For this review, use the dimensioned drawing (mm, ordinates from the lowest corner) and the shaded views. Round coordinates to 2 decimals unless told otherwise and drop trailing zeros. Write each loop counter-clockwise with the first axis right and the second up, starting at its lowest first coordinate (ties: lowest second). Pieces come first, ordered by that corner, then holes. Notation, with made-up numbers: M 47.5,46 L 99.5,46 A20 ccw 99.5,63 Z; hole C 74.25,72 d11. An arc over 180 degrees is marked long. One line per question, with ' | ' between items.
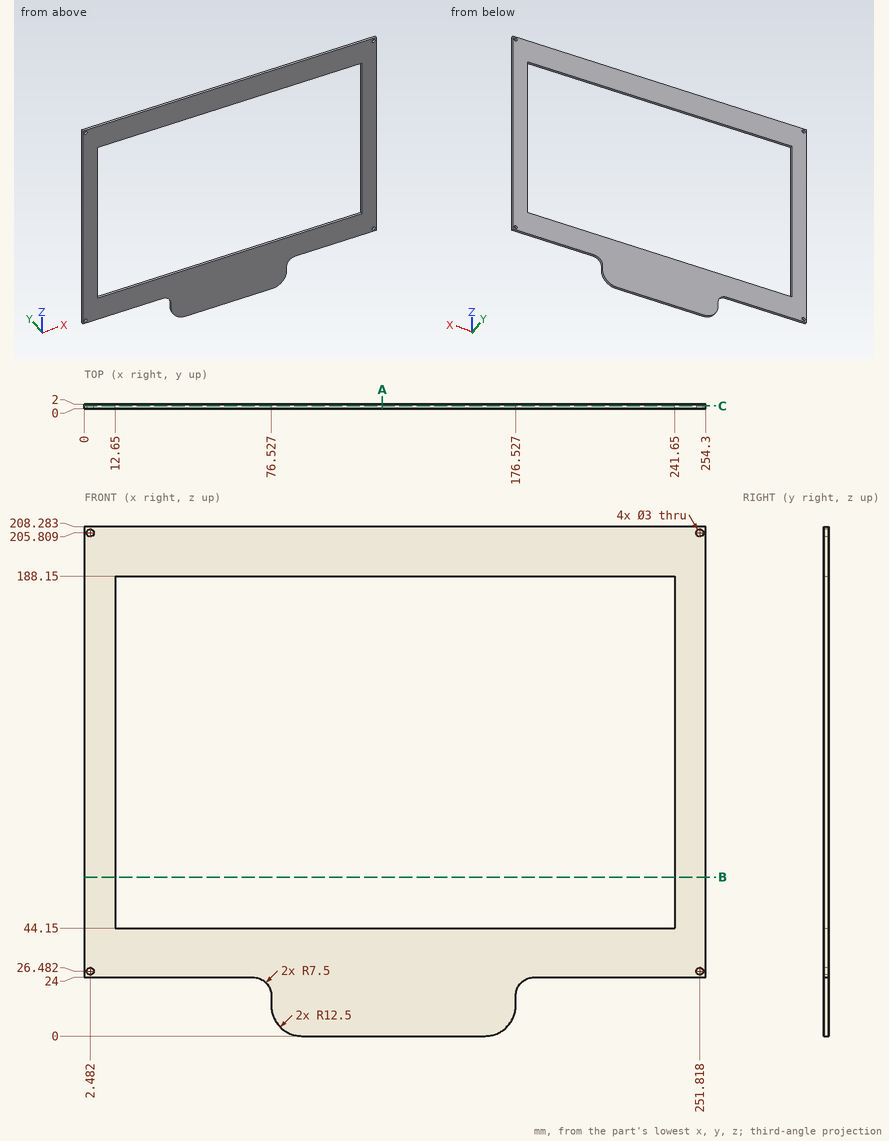
Item 1: Take a section at C-C (y = 1.2). Write out the cut boundary in (x, z).
Results:
outline: M 0,24 L 69.03,24 A7.5 cw 76.53,16.5 L 76.53,12.5 A12.5 ccw 89.03,0 L 164.03,0 A12.5 ccw 176.53,12.5 L 176.53,16.5 A7.5 cw 184.03,24 L 254.3,24 L 254.3,208.28 L 0,208.28 Z; hole C 2.48,26.48 d3; hole C 2.48,205.81 d3; hole M 12.65,44.15 L 241.65,44.15 L 241.65,188.15 L 12.65,188.15 Z; hole C 251.82,26.48 d3; hole C 251.82,205.81 d3
Item 2: To check wall thickness, follow line 1 along Z through (x, y) = (216, 0.8); line 2 along X through (y, z) = (1.25, 152); line 3 along Z through (x, y) = (131.5, 0.4). State the ranges of each line that lie inside material, in increasing order. Write a range as from..to.
Results:
line 1: 24..44.15, 188.15..208.28 | line 2: 0..12.65, 241.65..254.3 | line 3: 0..44.15, 188.15..208.28
Item 3: Insertion check: pin 1 Ø1 at (y, z) = (1, 15.5) entering from -X; pin 2 Ø0.6 at (x, y) = (214.5, 0.5) entering from -Z; pin 3 Ø0.6 at (x, y) = (175.5, 0.5) entering from -Z (1 decimal). Each pin has a flat end and moves straight along its axis. Give the tip position at first contact, or say it passes through.
Results:
pin 1: x = 76.53 | pin 2: z = 24 | pin 3: z = 6.9
Item 4: Take a section at B-B (z = 65). Write out the cut boundary in (x, y).
Results:
outline: M 0,0 L 12.65,0 L 12.65,2 L 0,2 Z; M 241.65,0 L 254.3,0 L 254.3,2 L 241.65,2 Z
Item 5: Take a section at A-A (x = 122). Write out the cut boundary in (y, z).
Results:
outline: M 0,0 L 2,0 L 2,44.15 L 0,44.15 Z; M 0,188.15 L 2,188.15 L 2,208.28 L 0,208.28 Z
